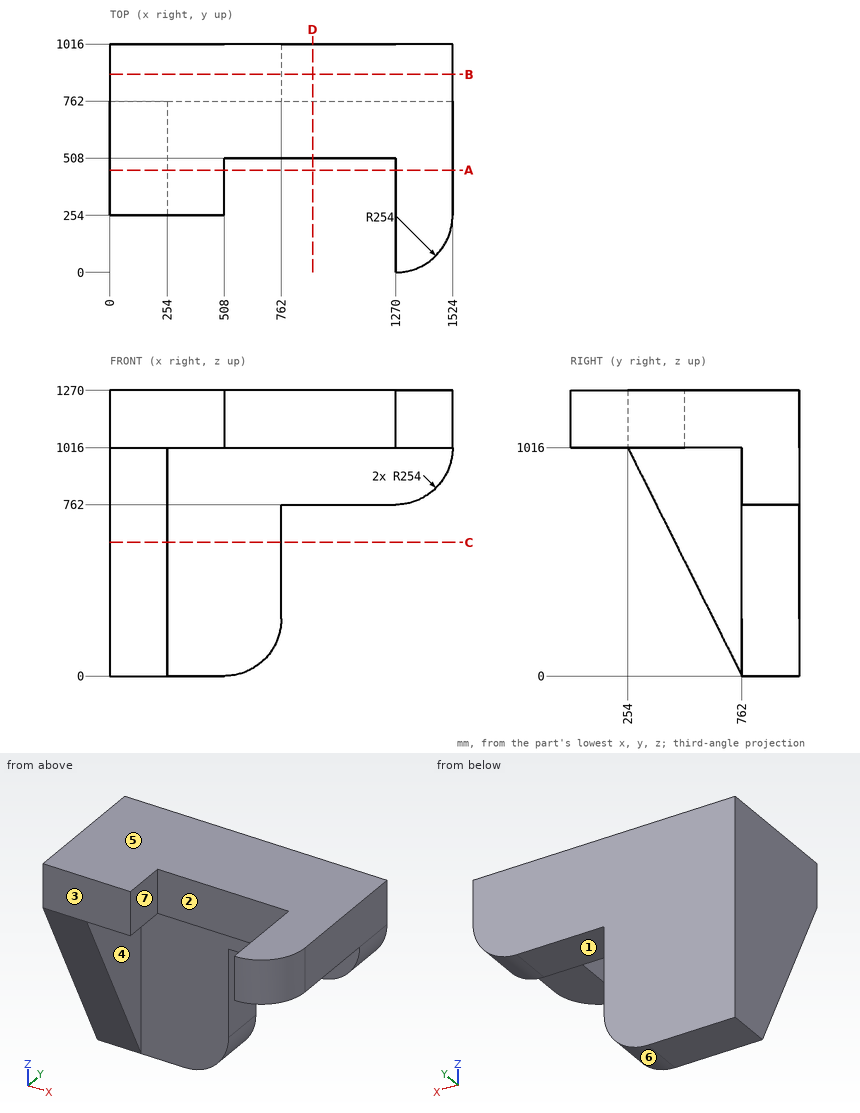
Design review of the part shown in the three views and the two pictorial views. Dimensions are in mm from the part's minimum x, y and z. A direction names the side the tool comes from. Round coordinates to 2 decimals unless told otherwise and drop trailing zeros. Loops run counter-clockwise (first coordinate to the right, second up) from the corner with the lowest first, then second, coordinate; pieces in that order, holes last. Notation, with made-up numbers: (40, 24) -> (81, 24) arc R16 cw to (81, 44) -> close; hole circle Ø10 at (-38, 47.5). An arc over 180 degrees is marked (long way). Return JSON: item names as keys, results as strings.
(1) Add section D-D on x = 901.5. Write out the cut boundary in (y, z), plus the area to 3 significant figures.
Solved:
{"outline": "(508, 1016) -> (762, 1016) -> (762, 762) -> (1016, 762) -> (1016, 1270) -> (508, 1270) -> close", "area": "194,000 mm2"}
(2) Add section B-B on y = 881. Write out the cut boundary in (x, z).
Solved:
{"outline": "(0, 0) -> (508, 0) arc R254 ccw to (762, 254) -> (762, 762) -> (1270, 762) arc R254 ccw to (1524, 1016) -> (1524, 1270) -> (0, 1270) -> close"}
(3) Add section A-A on y = 455.5. Write out the cut boundary in (x, z).
Solved:
{"outline": "(0, 613) -> (254, 613) -> (254, 1016) -> (508, 1016) -> (508, 1270) -> (0, 1270) -> close; (1270, 1016) -> (1524, 1016) -> (1524, 1270) -> (1270, 1270) -> close"}
(4) Add section C-C on z = 594. Write out the cut boundary in (x, y).
Solved:
{"outline": "(0, 465) -> (254, 465) -> (254, 762) -> (762, 762) -> (762, 1016) -> (0, 1016) -> close"}
(5) For pin 1 (3 mm diameter, centred on x = 1330.5, y = 162, fed in from -Z); pin 2 (1 mm diameter, centred on x = 242.5, z = 809.5, fed in from -Y); pin 3 (1.5 mm diameter, centred on x = 1031, y = 842.5, fed in from -Z), all flat-tipped, find the tip position at first contact; note any pin that passes through.
Solved:
{"pin 1": "z = 1016", "pin 2": "y = 357", "pin 3": "z = 762"}
(6) The part is to be moulded in two halves that separate along X. For the marked faces 5, 6 and 7, say which applies: released by +X, released by -X, zero draft, split by the parting line, or undercut.
Solved:
{"face 5": "zero draft", "face 6": "released by +X", "face 7": "undercut"}
(7) For line 1 (X direction, y = 860.5, z = 548); line 2 (Y direction, x = 564.5, z = 285.5); line 3 (Z direction, x = 804.5, y = 600), list the stretches that pass through material, from the lowest coordinate up.
Solved:
{"line 1": "0 to 762", "line 2": "762 to 1016", "line 3": "1016 to 1270"}
(8) For the marked faces 1, 2, 3 and 4, list the 3-axis set-ups (+Z, -Z, +X, -X, +Y, -Y) from which the entire face can be reached by the end or side of a thin tool; tool diameter is ignored.
Solved:
{"face 1": "-Z, +X, +Y, -Y", "face 2": "+Z, -Z, -Y", "face 3": "+Z, -Z, -X, -Y", "face 4": "-Z, +X, -Y"}
